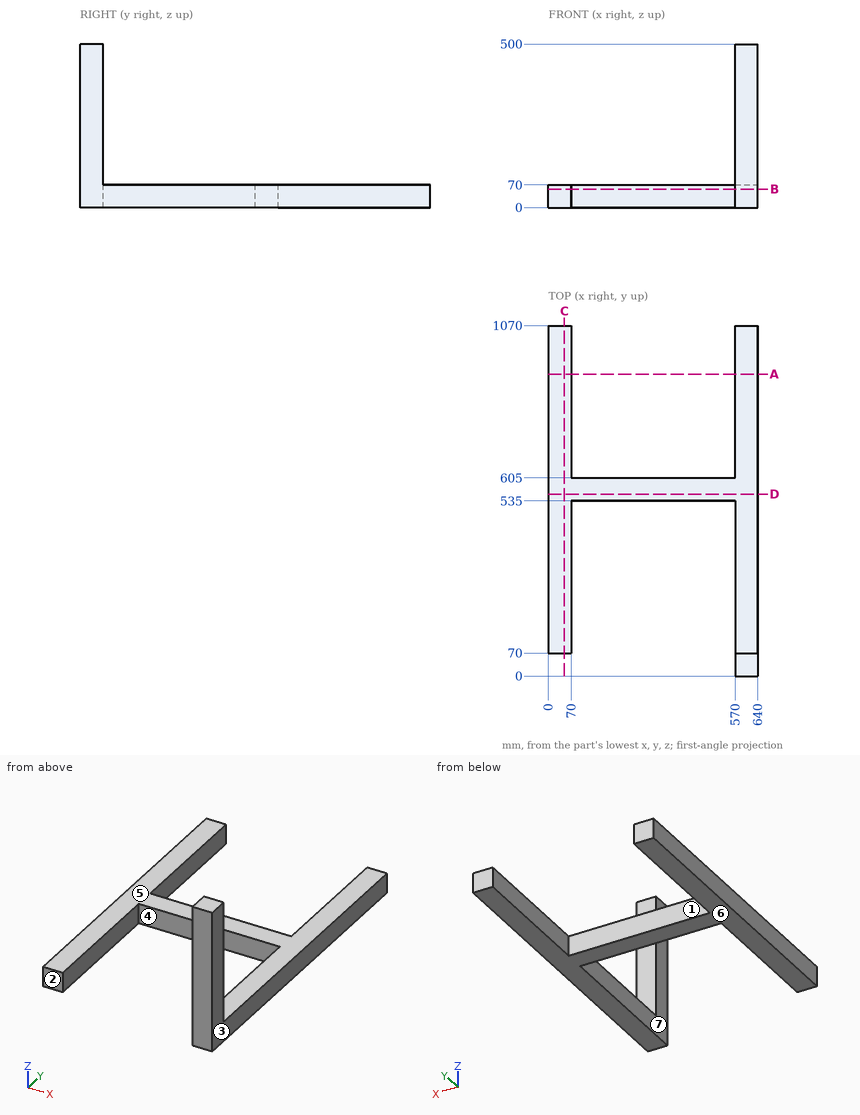
Here's the drawing with two shaded views (mm, measured from the low corner). I have some questions. A direction names the side the tool comes from. Coordinates: 2 decimals unless noted, no trailing zeros. Order: outer loops, then holes, each group sorted by start corner. A loop starts at its lowest first (then second) coordinate and runs counter-clockwise, first axis right, second up. Notation, with made-up numbers: (51.5, 1.25) -> (91.5, 1.25) arc R12 ccw to (91.5, 23.25) -> close; hole circle Ø9 at (-15.5, 35.5). An arc over 180 degrees is marked (long way). Write each question's results on one line, items separated by ' | '.
Item 1: I want a section at A-A, the plane y = 922. Write out the boundary of the cut face in (x, z).
Results are:
outline: (0, 0) -> (70, 0) -> (70, 70) -> (0, 70) -> close; (570, 0) -> (640, 0) -> (640, 70) -> (570, 70) -> close
Item 2: Which directions (+Z, -Z, +X, -X, +Y, -Y) give clear straight access to the entire face, cutting with the end or side of a thin tool? Please do the marked faces 5, 6 and 7.
Results are:
face 5: +Z, +X, -X, +Y | face 6: -Z, +X, -X, +Y, -Y | face 7: +Z, -Z, -Y
Item 3: I want a section at D-D, the plane y = 555.5. Write out the boundary of the cut face in (x, z).
Results are:
outline: (0, 0) -> (640, 0) -> (640, 70) -> (0, 70) -> close
Item 4: If we mould it in two halves opening along X, with no side actions, what happens to the marked faces 1, 2, 3 and 4? For each: +X half, -X half, draft (parallel to the pull), parting line (faces both ways), or undercut.
Results are:
face 1: undercut | face 2: draft | face 3: +X half | face 4: undercut
Item 5: I'm going to push flat-ended pins straight in: pin 1 Ø21 at (x, z) = (28.5, 22) entering from -Y; pin 2 Ø2 at (x, z) = (558.5, 69.5) entering from +Y. Where does each tip first touch, or does it pass through?
Results are:
pin 1: y = 70 | pin 2: y = 605
Item 6: I want a section at C-C, the plane x = 48.5. Write out the boundary of the cut face in (y, z).
Results are:
outline: (70, 0) -> (1070, 0) -> (1070, 70) -> (70, 70) -> close
Item 7: I want a section at B-B, the plane z = 56.5. Write out the boundary of the cut face in (x, y).
Results are:
outline: (0, 70) -> (70, 70) -> (70, 535) -> (570, 535) -> (570, 0) -> (640, 0) -> (640, 1070) -> (570, 1070) -> (570, 605) -> (70, 605) -> (70, 1070) -> (0, 1070) -> close
Item 8: If I drill on line 1 along Y through (x, z) = (591, 284); line 2 along X through (y, z) = (56, 265); line 3 along Y through (x, z) = (388.5, 57.5), over which ranges is the centre line in solid material (lowest first)?
Results are:
line 1: 0 to 70 | line 2: 570 to 640 | line 3: 535 to 605
